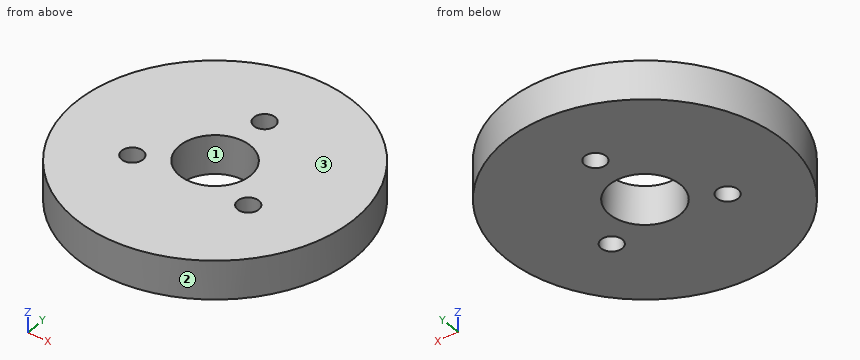
from build123d import *

# Parameters (mm, degrees)
SKETCH1_R           = 21.6
SKETCH1_R_2         = 5.5
BOSS_EXTRUDE1_DEPTH = 6
SKETCH2_R           = 1.65
CUT_EXTRUDE1_DEPTH  = 7


with BuildPart() as part:
    # Sketch1 → Boss-Extrude1 (new body)
    with BuildSketch(Plane.XY):
        Circle(SKETCH1_R)
        Circle(SKETCH1_R_2, mode=Mode.SUBTRACT)
    extrude(amount=BOSS_EXTRUDE1_DEPTH)

    # Sketch2 → Cut-Extrude1 (cut, through all)
    with BuildSketch(Plane.XY.offset(6)):
        with Locations((0, 10.45)):
            Circle(SKETCH2_R)
        with Locations((9.04996547, -5.225)):
            Circle(SKETCH2_R)
        with Locations((-9.04996547, -5.225)):
            Circle(SKETCH2_R)
    extrude(amount=-CUT_EXTRUDE1_DEPTH, mode=Mode.SUBTRACT)


solid = part.part
Design review of the part built by this model. Coordinates are the model's own, in mm. Face numbers are marked on the shaded views. Give positions to 0.01 mm unless a question says otherwise; leave off trailing zeros. Write each loop counter-clockwise with the first axis right and the second up, starting at its lowest first coordinate (ties: lowest second). Pieces come first, ordered by that corner, then holes. Notation, with made-up numbers: M -23.75,-9.5 L 15.25,-9.5 A36 cw 15.25,24.5 Z; hole C -19.5,27 d1. An arc over 180 degrees is marked long. Answer as a JSON object with one key per item and string values. Group by question number.
1) We need section B-B (x = 0). Give the boundary of the cut face in (y, z), and give its area (3 significant figures).
2) We need section D-D (z = 1.25). Give the boundary of the cut face in (x, y) (3 decimals).
3) We need section A-A (y = 0). Give the boundary of the cut face in (x, z).
4) For line 1 along Y through (x, z) = (0, 1.65); line 2 along X through (y, z) = (-4, 2.65); line 3 along X through (y, z) = (-5, 3.25), list the stretches that pass through material, from the lowest coordinate up.
5) Mouldability with a two-part tool opening along X and no side actions: class the marked faces 1, 2 and 3 as released by +X, released by -X, zero draft, split by the parting line, or undercut.
6) Clearance check with flat-ended pins moving along their axes: pin 1 Ø1 at (x, z) = (-2, 4) entering from +Y; pin 2 Ø2 at (y, z) = (-7, 3) entering from -X. State where each tip first meets the part, or that it passes through.
7) We need section C-C (x = -9). Give the boundary of the cut face in (y, z), and give its area (3 significant figures).
Answer key:
{
 "1": {"outline": "M -21.6,0 L -5.5,0 L -5.5,6 L -21.6,6 Z; M 5.5,0 L 8.8,0 L 8.8,6 L 5.5,6 Z; M 12.1,0 L 21.6,0 L 21.6,6 L 12.1,6 Z", "area": "173 mm²"},
 "2": {"outline": "C 0,0 d43.2; hole C -9.05,-5.225 d3.3; hole C 0,0 d11; hole C 0,10.45 d3.3; hole C 9.05,-5.225 d3.3"},
 "3": {"outline": "M -21.6,0 L -5.5,0 L -5.5,6 L -21.6,6 Z; M 5.5,0 L 21.6,0 L 21.6,6 L 5.5,6 Z"},
 "4": {"line 1": "y = -21.6 to -5.5, 5.5 to 8.8, 12.1 to 21.6", "line 2": "x = -21.23 to -10.16, -7.94 to -3.77, 3.77 to 7.94, 10.16 to 21.23", "line 3": "x = -21.01 to -10.68, -7.42 to -2.29, 2.29 to 7.42, 10.68 to 21.01"},
 "5": {"face 1": "undercut", "face 2": "split by the parting line", "face 3": "zero draft"},
 "6": {"pin 1": "stops at y = 21.55", "pin 2": "stops at x = -20.75"},
 "7": {"outline": "M -19.64,0 L -6.87,0 L -6.87,6 L -19.64,6 Z; M -3.58,0 L 19.64,0 L 19.64,6 L -3.58,6 Z", "area": "216 mm²"}
}
